```python
from build123d import *

# Parameters (mm, degrees)
F0_W     = 101.6
F0_H     = 101.6
F0_R     = 31.75
F1_DEPTH = 38.1
F0_W_2   = 152.4
F0_H_2   = 152.4
F2_DEPTH = 50.8


with BuildPart() as f1:
    # F0 (on Front) → F1 (new body)
    with BuildSketch(Plane.XZ):
        Rectangle(F0_W, F0_H)
        Circle(F0_R, mode=Mode.SUBTRACT)
    extrude(amount=-F1_DEPTH)

    # F0 (on Front) → F2 (join)
    with BuildSketch(Plane.XZ):
        with Locations((2.284581, 0)):
            Rectangle(F0_W_2, F0_H_2)
        Rectangle(F0_W, F0_H, mode=Mode.SUBTRACT)
        Rectangle(F0_W, F0_H)
        Circle(F0_R, mode=Mode.SUBTRACT)
    extrude(amount=F2_DEPTH)


solid = f1.part
```
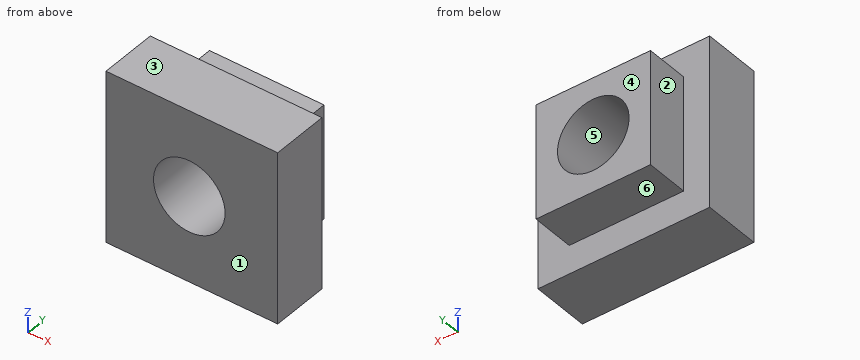
Build history of the part. All positions in model axes, mm. Face numbers are marked on the shaded views. A direction names the side the tool comes from. Round coordinates to 2 decimals unless told otherwise and drop trailing zeros. Write each loop counter-clockwise with the first axis right and the second up, starting at its lowest first coordinate (ties: lowest second). Pieces come first, ordered by that corner, then holes. Notation, with made-up numbers: (28.5, 37.5) -> (83.5, 37.5) arc R10 cw to (83.5, 45.5) -> close; hole circle Ø2 at (53.25, 89.25). An arc over 180 degrees is marked (long way). Put each result on its own line as item: value.
Item 1: Flat gauge pins, fed straight in: P1, Ø3, axis at x = -32, z = 54, coming from the +Y side; P2, Ø19, axis at x = -21.5, y = 23, coming from the -Z side; P3, Ø11.5, axis at y = 10, z = 9.5, coming from the -X side. Where does each tip first touch, or does it go through?
Here are the results:
P1: stops at y = 0
P2: stops at z = -50.8
P3: stops at x = -50.8
Item 2: Tool access for the marked faces 1 and 2: list every direction of +Z, -Z, +X, -X, +Y, -Y with a clear straight run to the whole face (end or side of a thin tool).
Here are the results:
face 1: +Z, -Z, +X, -X, -Y
face 2: +Z, -Z, -X, +Y
Item 3: Wall check: probe 1 along Z at (x, y) = (1, 34); probe 2 along Z at (x, y) = (-17, 31); probe 3 along X at (y, z) = (-4.5, -5). Give the ranges that are in metal, low to high. Write a range as from..to.
Here are the results:
probe 1: z = -50.8..-31.73, 31.73..50.8
probe 2: z = -50.8..-26.82, 26.82..50.8
probe 3: x = -73.92..-31.35, 31.35..78.48
Item 4: Slice it at C-C, the plane x = 0. Give the cut face in (y, z).
Here are the results:
outline: (-50.8, -76.2) -> (0, -76.2) -> (0, -50.8) -> (38.1, -50.8) -> (38.1, -31.75) -> (-50.8, -31.75) -> close; (-50.8, 31.75) -> (38.1, 31.75) -> (38.1, 50.8) -> (0, 50.8) -> (0, 76.2) -> (-50.8, 76.2) -> close
Item 5: Slice it at B-B, the plane z = 0. Give the cut face in (x, y).
Here are the results:
outline: (-73.92, -50.8) -> (-31.75, -50.8) -> (-31.75, 38.1) -> (-50.8, 38.1) -> (-50.8, 0) -> (-73.92, 0) -> close; (31.75, -50.8) -> (78.48, -50.8) -> (78.48, 0) -> (50.8, 0) -> (50.8, 38.1) -> (31.75, 38.1) -> close
Item 6: Slice it at A-A, the plane y = 21.5. Give the cut face in (x, z), plus the area to 3 significant figures.
Here are the results:
outline: (-50.8, -50.8) -> (50.8, -50.8) -> (50.8, 50.8) -> (-50.8, 50.8) -> close; hole circle Ø63.5 at (0, 0)
area: 7,160 mm^2
Item 7: Two-plate mould, pull along Z, no slides. Class the marked faces 3, 4, 5 and 6: pulls with the +Z half, pulls with the -Z half, needs draft (parallel to the pull), parting line crosses it, or undercut.
Here are the results:
face 3: pulls with the +Z half
face 4: needs draft
face 5: undercut
face 6: pulls with the -Z half
Item 8: Slice it at D-D, the plane z = -37.5. Give the cut face in (x, y).
Here are the results:
outline: (-73.92, -50.8) -> (78.48, -50.8) -> (78.48, 0) -> (50.8, 0) -> (50.8, 38.1) -> (-50.8, 38.1) -> (-50.8, 0) -> (-73.92, 0) -> close
